CAD build for the part. Positions are in the model's coordinates, mm. A direction names the side the tool comes from. Round coordinates to 2 decimals unless told otherwise and drop trailing zeros. Order: outer loops, then holes, each group sorted by start corner. A loop starts at its lowest first (then second) coordinate and runs counter-clockwise, first axis right, second up. Notation, with made-up numbers: M 41.5,18.25 L 45.5,18.25 A22 cw 45.5,24.25 Z; hole C -9.5,65.25 d1. An arc over 180 degrees is marked long. Answer as a JSON object with one key per item and string values. Group by question number.
Autodesk Inventor part; units mm, degrees
ref_plane "YZ Plane" through (0, 0, 0) normal (1, 0, 0) x (0, 1, 0)
ref_plane "XZ Plane" through (0, 0, 0) normal (0, 1, 0) x (-1, 0, 0)
ref_plane "XY Plane" through (0, 0, 0) normal (0, 0, 1) x (1, 0, 0)
sketch "Sketch1" plane through (0, 0, 0) normal (0, 0, 1) x (1, 0, 0)
  circle A0 centre (-21, 1.215) radius 1.4
  circle A1 centre (21, 1.215) radius 1.4
  arc A2 (24.9, 3.115) -> (22.9, 5.115) centre (22.9, 3.115) ccw
  line L0 (22.9, 5.115) -> (-22.9, 5.115)
  arc A3 (-22.9, 5.115) -> (-24.9, 3.115) centre (-22.9, 3.115) ccw
  line L1 (-24.9, 3.115) -> (-24.9, -5.115)
  line L2 (-24.9, -5.115) -> (-22.8395, -5.115)
  line L3 (24.9, -5.115) -> (24.9, 3.115)
  arc A4 (22.9, -44.685) -> (24.9, -42.685) centre (22.9, -42.685) ccw
  line L4 (24.9, -42.685) -> (24.9, -36.885)
  line L5 (24.9, -36.885) -> (17.1, -36.885)
  line L6 (17.1, -36.885) -> (17.1, -44.685)
  line L7 (17.1, -44.685) -> (22.9, -44.685)
  circle A5 centre (21, -40.785) radius 1.4
  arc A6 (-24.9, -42.685) -> (-22.9, -44.685) centre (-22.9, -42.685) ccw
  line L8 (-22.9, -44.685) -> (-17.1, -44.685)
  line L9 (-17.1, -44.685) -> (-17.1, -36.885)
  line L10 (-17.1, -36.885) -> (-24.9, -36.885)
  line L11 (-24.9, -36.885) -> (-24.9, -42.685)
  circle A7 centre (-21, -40.785) radius 1.4
  line L12 (24.9, 5.115) -> (-24.9, 5.115)
  line L13 (-24.9, 5.115) -> (-24.9, -44.685)
  line L14 (-24.9, -44.685) -> (24.9, -44.685)
  line L15 (24.9, -44.685) -> (24.9, 5.115)
  line L16 (17.1, -2.685) -> (-17.1, -2.685)
  line L17 (-17.1, -2.685) -> (-17.1, -36.885)
  line L18 (-17.1, -36.885) -> (17.1, -36.885)
  line L19 (17.1, -36.885) -> (17.1, -2.685)
  line L20 (17.1, -36.885) -> (17.1, -44.685)
  line L21 (-17.1, -36.885) -> (-17.1, -44.685)
  circle A8 centre (0, 1.415) radius 1.4
  arc A9 (-18.2605, -5.115) -> (-22.8395, -5.115) centre (-20.55, -5.335) ccw
  arc A10 (22.8395, -5.115) -> (18.2605, -5.115) centre (20.55, -5.335) ccw
  circle A11 centre (14.45, 0.765) radius 2.3
  circle A12 centre (-14.45, 0.765) radius 2.3
  line L22 (-18.2605, -5.115) -> (18.2605, -5.115)
  line L23 (22.8395, -5.115) -> (24.9, -5.115)
  point P0 (0, 0)
  point P1 (-20.55, -5.335)
  point P2 (20.55, -5.335)
  point P3 (-20.55, -5.335)
  point P4 (20.55, -5.335)
  point P5 (-20.55, -5.335)
  point P6 (20.55, -5.335)
  dimension "d0" = 7.8
extrude "Extrusion1" add sketch "Sketch1" along normal blind 8 contours L3 L23 A10 L22 L19 L16 L17 A9 L2 L1 A3 L0 A2 | L15 L5 L19 L22 A10 L23 | L4 A4 L7 L6 L5 | L2 A9 L22 L17 L10 L13 | L9 L8 A6 L11 L10 | A8 | A11 | A12
sketch "Sketch2" plane through (0, 0, 8) normal (0, 0, 1) x (1, 0, 0)
  circle A0 centre (0, 1.715) radius 1.4
  line L0 (22.9, 5.115) -> (-22.9, 5.115)
  point P0 (0, 0)
  dimension "d3" = 2.8
  dimension "d4" = 3.4
extrude "Extrusion2" cut sketch "Sketch2" against normal blind 8
ref_plane "Arbeitsebene1" through (15.3065, -4.4785, 13.1) normal (0, 0, 1) x (0, 1, 0)
sketch "Skizze3" plane through (15.3065, -4.4785, 13.1) normal (0, 0, 1) x (0, 1, 0)
  line L0 (-0.7065, 32.7565) -> (-31.2065, 32.7565)
  arc A0 (1.2935, 30.7565) -> (-0.7065, 32.7565) centre (-0.7065, 30.7565) ccw
  line L1 (1.2935, 30.7565) -> (1.2935, 0.2565)
  arc A1 (-0.7065, -1.7435) -> (1.2935, 0.2565) centre (-0.7065, 0.2565) ccw
  line L2 (-0.7065, -1.7435) -> (-31.2065, -1.7435)
  arc A2 (-33.2065, 0.2565) -> (-31.2065, -1.7435) centre (-31.2065, 0.2565) ccw
  line L3 (-33.2065, 0.2565) -> (-33.2065, 30.7565)
  arc A3 (-31.2065, 32.7565) -> (-33.2065, 30.7565) centre (-31.2065, 30.7565) ccw
  line L4 (-38.9565, -9.4935) -> (-20.9565, -9.4935)
  arc A4 (7.0435, -9.4935) -> (9.0435, -7.4935) centre (7.0435, -7.4935) ccw
  line L5 (9.0435, 10.5065) -> (9.0435, -7.4935)
  line L6 (9.0435, 10.5065) -> (10.195, 10.5065)
  arc A5 (10.6845, 10.1086) -> (10.195, 10.5065) centre (10.195, 10.0065) ccw
  arc A6 (10.6845, 10.1086) -> (14.5435, 10.5065) centre (12.5935, 10.5065) ccw
  line L7 (14.5435, 10.5065) -> (14.5435, 20.6065)
  line L8 (9.0435, 38.5065) -> (9.0435, 20.5065)
  arc A7 (9.0435, 38.5065) -> (7.0435, 40.5065) centre (7.0435, 38.5065) ccw
  line L9 (-21.0689, 40.5065) -> (-38.9565, 40.5065)
  line L10 (7.0435, 40.5065) -> (-10.8565, 40.5065)
  arc A8 (-38.9565, 40.5065) -> (-40.9565, 38.5065) centre (-38.9565, 38.5065) ccw
  line L11 (-40.9565, 20.6065) -> (-40.9565, 38.5065)
  line L12 (-40.9565, -7.4935) -> (-40.9565, 10.3942)
  arc A9 (-40.9565, -7.4935) -> (-38.9565, -9.4935) centre (-38.9565, -7.4935) ccw
  line L13 (-20.9565, -9.4935) -> (-20.9565, -10.645)
  arc A10 (-21.3545, -11.1345) -> (-20.9565, -10.645) centre (-21.4565, -10.645) ccw
  arc A11 (-21.3545, -11.1345) -> (-20.9565, -14.9935) centre (-20.9565, -13.0435) ccw
  line L14 (-20.9565, -14.9935) -> (-10.8565, -14.9935)
  circle A12 centre (-15.9565, -5.8535) radius 1.6
  circle A13 centre (5.4035, 15.5065) radius 1.6
  line L15 (-21.0689, 39.3752) -> (-21.0689, 40.5065)
  line L16 (-40.9565, 20.6065) -> (-39.8237, 20.6065)
  arc A14 (-39.8237, 20.6065) -> (-39.429, 20.9412) centre (-39.8237, 21.0065) ccw
  arc A15 (-35.3565, 20.6065) -> (-39.429, 20.9412) centre (-37.4065, 20.6065) ccw
  line L17 (-35.3565, 20.6065) -> (-35.3565, 10.5065)
  arc A16 (-39.4194, 10.1183) -> (-35.3565, 10.5065) centre (-37.4065, 10.5065) ccw
  arc A17 (-39.4194, 10.1183) -> (-39.8252, 10.3942) centre (-39.7609, 10.0524) ccw
  line L18 (-39.8252, 10.3942) -> (-40.9565, 10.3942)
  arc A18 (-10.8565, -14.9935) -> (-10.5382, -11.1196) centre (-10.8565, -13.0435) ccw
  arc A19 (-10.9565, -10.6263) -> (-10.5382, -11.1196) centre (-10.4565, -10.6263) ccw
  line L19 (-10.9565, -10.6263) -> (-10.9565, -9.4935)
  line L20 (-10.9565, -9.4935) -> (7.0435, -9.4935)
  arc A20 (14.5435, 20.6065) -> (10.6696, 20.9249) centre (12.5935, 20.6065) ccw
  arc A21 (10.1763, 20.5065) -> (10.6696, 20.9249) centre (10.1763, 21.0065) ccw
  line L21 (10.1763, 20.5065) -> (9.0435, 20.5065)
  line L22 (-10.8565, 40.5065) -> (-10.8565, 39.3737)
  arc A22 (-10.8565, 39.3737) -> (-10.5218, 38.979) centre (-10.4565, 39.3737) ccw
  arc A23 (-10.8565, 34.9065) -> (-10.5218, 38.979) centre (-10.8565, 36.9565) ccw
  line L23 (-10.8565, 34.9065) -> (-20.9565, 34.9065)
  arc A24 (-21.3448, 38.9694) -> (-20.9565, 34.9065) centre (-20.9565, 36.9565) ccw
  arc A25 (-21.3448, 38.9694) -> (-21.0689, 39.3752) centre (-21.4107, 39.3109) ccw
  circle A26 centre (4.0435, -4.4935) radius 2.45
  circle A27 centre (-1.4565, -5.2935) radius 2.3
  circle A28 centre (4.8435, 1.0065) radius 2.3
  circle A29 centre (4.8435, 30.0065) radius 2.3
  circle A30 centre (-1.4565, 36.3065) radius 2.3
  circle A31 centre (4.0435, 35.5065) radius 2.45
  circle A32 centre (-36.7565, 1.0065) radius 2.3
  circle A33 centre (-30.4565, -5.2935) radius 2.3
  circle A34 centre (-35.9565, -4.4935) radius 2.45
  circle A35 centre (-36.7565, 30.0065) radius 2.3
  circle A36 centre (-30.4565, 36.3065) radius 2.3
  circle A37 centre (-35.9565, 35.5065) radius 2.45
  point P0 (4.4785, 15.3065)
hole "Bohrung1" [suppressed]
sketch "Skizze4" plane through (0, 0, 8) normal (0, 0, 1) x (1, 0, 0)
  circle A0 centre (0, 1.715) radius 1.4
  line L0 (17.1, -2.685) -> (17.1, -44.685)
  line L1 (17.1, -44.685) -> (22.9, -44.685)
  arc A1 (22.9, -44.685) -> (24.9, -42.685) centre (22.9, -42.685) ccw
  line L2 (24.9, -42.685) -> (24.9, 3.115)
  arc A2 (24.9, 3.115) -> (22.9, 5.115) centre (22.9, 3.115) ccw
  line L3 (22.9, 5.115) -> (-22.9, 5.115)
  arc A3 (-22.9, 5.115) -> (-24.9, 3.115) centre (-22.9, 3.115) ccw
  line L4 (-24.9, 3.115) -> (-24.9, -42.685)
  arc A4 (-24.9, -42.685) -> (-22.9, -44.685) centre (-22.9, -42.685) ccw
  line L5 (-22.9, -44.685) -> (-17.1, -44.685)
  line L6 (-17.1, -44.685) -> (-17.1, -2.685)
  line L7 (-17.1, -2.685) -> (17.1, -2.685)
  circle A5 centre (-21, -40.785) radius 1.4
  circle A6 centre (21, -40.785) radius 1.4
  circle A7 centre (-21, 1.215) radius 1.4
  circle A8 centre (21, 1.215) radius 1.4
  point P0 (0, 0)
hole "Bohrung2" at (-21, 1.215, 8) at (21, 1.215, 8) at (21, -40.785, 8) at (-21, -40.785, 8) direction (0, 0, -1) diameter 3 end through all counterbore diameter 6.5 counterbore depth 4
properties part number "00_Linear_Stage_NEMA11_Mount_Lid"
Item 1: 3-axis set-ups, long thin cutter, end or side, ignore diameter. For faces 4 (the face through (-17.1, -23, 4)), 5 (the face through (-17.827, 1.92, 5.972)), 6 (the face through (19.513, 1.41, 1.972)): which of +Z, -Z, +X, -X, +Y, -Y reach the whole face in a straight line?
Item 2: Cut at A-A, the plane x = 21. Give the cut face in (y, z) (3 decimals), and give its area (3 significant figures).
Item 3: Drill centre lines: line 1 (X direction, y = -11.5, z = 1.5); line 2 (X direction, y = -38, z = 5); line 3 (Y direction, x = 21, z = 2.4) (3 decimals). Where is each one in solid material? Low to high. Write a range as [from, to].
Item 4: Flat gauge pins, fed straight in: pin 1 Ø2.5 at (x, y) = (0, 1.715) entering from -Z; pin 2 Ø4 at (x, z) = (-4.5, 3) entering from -Y (3 decimals); pin 3 Ø3 at (x, y) = (21, -0.5) entering from +Z. Where does each tip first touch, or does it go through?
Item 5: Cut at C-C, the plane x = 0. Give the cut face in (y, z) (3 decimals), and give its area (3 significant figures).
Item 6: Cut at B-B, the plane y = -10. Give the cut face in (x, z).
Item 7: Two-plate mould, pull along Y, no slides. Class faces 1 (the face through (19.5, -41.5, 4)), 2 (the face through (0, -2.685, 4)), 3 (the face through (0, 5.115, 4)): +Y half, -Y half, draft (parallel to the pull), parting line (faces both ways), or undercut.
Item 8: Cut at D-D, the plane z = 5.25. Give the cut face in (x, y) (3 decimals), and give its area (3 significant figures).
Response values:
{
 "1": {"face 4": "+Z, -Z, -Y", "face 5": "+Z", "face 6": "+Z, -Z"},
 "2": {"outline": "M -44.685,0 L -42.285,0 L -42.285,4 L -44.035,4 L -44.035,8 L -44.685,8 Z; M -39.285,0 L -0.285,0 L -0.285,4 L -2.035,4 L -2.035,8 L -37.535,8 L -37.535,4 L -39.285,4 Z; M 2.715,0 L 5.115,0 L 5.115,8 L 4.465,8 L 4.465,4 L 2.715,4 Z", "area": "322 mm^2"},
 "3": {"line 1": "[-24.9, -17.1], [17.1, 24.9]", "line 2": "[-24.9, -22.68], [-19.32, -17.1], [17.1, 19.32], [22.68, 24.9]", "line 3": "[-44.685, -42.285], [-39.285, -0.285], [2.715, 5.115]"},
 "4": {"pin 1": "through", "pin 2": "y = -2.685", "pin 3": "z = 4"},
 "5": {"outline": "M -2.685,0 L 0.315,0 L 0.315,8 L -2.685,8 Z; M 3.115,0 L 5.115,0 L 5.115,8 L 3.115,8 Z", "area": "40.0 mm^2"},
 "6": {"outline": "M -24.9,0 L -17.1,0 L -17.1,8 L -24.9,8 Z; M 17.1,0 L 24.9,0 L 24.9,8 L 17.1,8 Z"},
 "7": {"face 1": "undercut", "face 2": "-Y half", "face 3": "+Y half"},
 "8": {"outline": "M -24.9,-42.685 A2 ccw -22.9,-44.685 L -17.1,-44.685 L -17.1,-2.685 L 17.1,-2.685 L 17.1,-44.685 L 22.9,-44.685 A2 ccw 24.9,-42.685 L 24.9,3.115 A2 ccw 22.9,5.115 L -22.9,5.115 A2 ccw -24.9,3.115 Z; hole C -21,-40.785 d6.5; hole C -21,1.215 d6.5; hole C 0,1.715 d2.8; hole C 21,-40.785 d6.5; hole C 21,1.215 d6.5", "area": "901 mm^2"}
}
